Verification items for the finished model (mm, model axes). Face numbers are marked on the shaded views. A direction names the side the tool comes from. Round coordinates to 2 decimals unless told otherwise and drop trailing zeros. Write each loop counter-clockwise with the first axis right and the second up, starting at its lowest first coordinate (ties: lowest second). Pieces come first, ordered by that corner, then holes. Notation, with made-up numbers: M 64.25,-32.75 L 94.25,-32.75 A24 ccw 94.25,-19.75 Z; hole C 87.25,-36.75 d5. An arc over 180 degrees is marked long. One line per item, written item: value. Start each with the question number.
Item 1: Thickness scan on probe 1 along Z at (x, y) = (13, 0.15); probe 2 along X at (y, z) = (2.15, -0.1); probe 3 along Y at (x, z) = (7, -2.35). Record the ranges inside material, lowest first. Write a range as from..to.
Item 2: Gauge pin test, flat ends, axial feed: pin 1 (3 mm diameter, centred on x = 18.5, y = -2, fed in from +Z); pin 2 (2.5 mm diameter, centred on x = 28.5, z = -0.5, fed in from +Y); pin 3 (1.2 mm diameter, centred on y = 2.5, z = 0.5, fed in from +X). Record the tip position at first contact, or that the pin passes through.
Item 3: Section check A-A, the plane z = 0. Record the cut outline in (x, y).
Item 4: Section check B-B, the plane x = 5.5. Record the cut outline in (y, z).
Item 5: Section check D-D, the plane x = 11. Record the cut outline in (y, z), then the cut area to 3 significant figures.
Item 6: Section check C-C, the plane y = 0.9. Record the cut outline in (x, z), then the cut area to 3 significant figures.
Item 7: Tool access check on the marked faces 1, 2, 3, 4 and 5. Record the directions out of +Z, -Z, +X, -X, +Y, -Y that give a thin tool (end or side, any length) a straight path to the whole face; none if there is none.
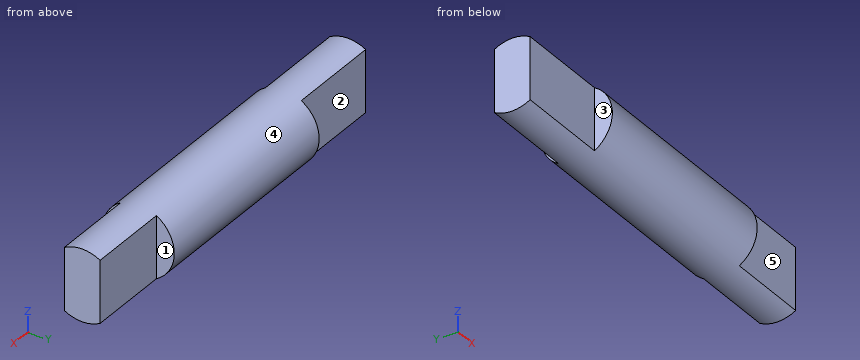
from build123d import *

# Parameters (mm, degrees)
SKETCH1_R           = 3
BOSS_EXTRUDE1_DEPTH = 33
CUT_EXTRUDE1_DEPTH  = 8
CUT_EXTRUDE2_START  = -7
CUT_EXTRUDE2_DEPTH  = 7


with BuildPart() as part:
    # Sketch1 → Boss-Extrude1 (new body)
    with BuildSketch(Plane(origin=(0, 0, 0), x_dir=(0, 0, -1), z_dir=(1, 0, 0))):
        Circle(SKETCH1_R)
    extrude(amount=BOSS_EXTRUDE1_DEPTH)

    # Sketch2 → Cut-Extrude1 (cut)
    with BuildSketch(Plane.ZY):
        with BuildLine():
            Line((-2.598076211, 1.5), (2.598076211, 1.5))
            ThreePointArc((2.598076211, 1.5), (0, 3), (-2.598076211, 1.5))
        make_face()
        with BuildLine():
            Line((-2.598076211, -1.5), (2.598076211, -1.5))
            ThreePointArc((2.598076211, -1.5), (0, -3), (-2.598076211, -1.5))
        make_face()
    extrude(amount=-CUT_EXTRUDE1_DEPTH, mode=Mode.SUBTRACT)

    # Sketch3 → Cut-Extrude2 (cut)
    with BuildSketch(Plane(origin=(33, 0, 0), x_dir=(0, 0, -1), z_dir=(1, 0, 0)).offset(CUT_EXTRUDE2_START)):
        with BuildLine():
            Line((-2.598076211, 1.5), (2.598076211, 1.5))
            ThreePointArc((2.598076211, 1.5), (0, 3), (-2.598076211, 1.5))
        make_face()
        with BuildLine():
            Line((-2.598076211, -1.5), (2.598076211, -1.5))
            ThreePointArc((2.598076211, -1.5), (0, -3), (-2.598076211, -1.5))
        make_face()
    extrude(amount=CUT_EXTRUDE2_DEPTH, mode=Mode.SUBTRACT)


solid = part.part
Response values:
1. probe 1: z = -3..3
1. probe 2: x = 8..26
1. probe 3: y = -1.5..1.5
2. pin 1: stops at z = 2.96
2. pin 2: stops at y = 1.5
2. pin 3: stops at x = 26
3. outline: M 0,-1.5 L 8,-1.5 L 8,-3 L 26,-3 L 26,-1.5 L 33,-1.5 L 33,1.5 L 26,1.5 L 26,3 L 8,3 L 8,1.5 L 0,1.5 Z
4. outline: M -1.5,-2.6 A3 ccw 1.5,-2.6 L 1.5,2.6 A3 ccw -1.5,2.6 Z
5. outline: C 0,0 d6
5. area: 28.3 mm2
6. outline: M 0,-2.86 L 33,-2.86 L 33,2.86 L 0,2.86 Z
6. area: 189 mm2
7. face 1: +Z, -Z, +X, +Y
7. face 2: +Z, -Z, -X, +Y
7. face 3: +Z, -Z, -X, -Y
7. face 4: +X, -X
7. face 5: +Z, -Z, +X, -Y
